Verification items for the finished model (mm, model axes). Face numbers are marked on the shaded views. A direction names the side the tool comes from. Round coordinates to 2 decimals unless told otherwise and drop trailing zeros. Write each loop counter-clockwise with the first axis right and the second up, starting at its lowest first coordinate (ties: lowest second). Pieces come first, ordered by that corner, then holes. Notation, with made-up numbers: M -6,49 L 40,49 A18 cw 40,61 Z; hole C 57.25,71 d7. An arc over 180 degrees is marked long. One line per item, written item: value. Start each with the question number.
Item 1: Gauge pin test, flat ends, axial feed: pin 1 (1.5 mm diameter, centred on y = 6.5, z = 4, fed in from -X); pin 2 (17 mm diameter, centred on x = 0, y = 0, fed in from -Z); pin 3 (4 mm diameter, centred on x = -6, z = 1.5, fed in from +Y). Record the tip position at first contact, or that the pin passes through.
Item 2: Thickness scan on probe 1 along Y at (x, z) = (0, 2.5) (3 decimals); probe 2 along Z at (x, y) = (11, 7.75); probe 3 along Y at (x, z) = (0, -1.85) (3 decimals). Record the ranges inside material, lowest first. Write a range as from..to.
Item 3: Tool access check on the marked faces 1, 2 and 3. Record the directions out of +Z, -Z, +X, -X, +Y, -Y that give a thin tool (end or side, any length) a straight path to the whole face; none if there is none.
Item 4: Section check C-C, the plane z = 2.75. Record the cut outline in (x, y) (3 decimals).
Autodesk Inventor part; units mm, degrees
ref_plane "YZ Plane" through (0, 0, 0) normal (1, 0, 0) x (0, 1, 0)
ref_plane "XZ Plane" through (0, 0, 0) normal (0, 1, 0) x (-1, 0, 0)
ref_plane "XY Plane" through (0, 0, 0) normal (0, 0, 1) x (1, 0, 0)
sketch "Sketch1" plane through (0, 0, 0) normal (0, 0, 1) x (1, 0, 0)
  circle A0 centre (0, 0) radius 9.525
  circle A1 centre (0, 0) radius 12.7
  circle A2 centre (0, 0) radius 14.2875
  dimension "d0" = 19.05
  dimension "d1" = 25.4
  dimension "d2" = 28.575
extrude "Extrusion1" add sketch "Sketch1" along normal blind 4.7625 contours A1
extrude "Extrusion2" add sketch "Sketch1" against normal blind 1.5875 contours A1 | A2
chamfer "Chamfer1" distance 0.254 angle 45 4 edges at (-12.7, 0, 4.7625) (-9.525, 0, 4.7625) (-14.2875, 0, 0) (-14.2875, 0, -1.5875)
sketch "Sketch2" plane through (0, 0, -1.5875) normal (0, 0, -1) x (-1, 0, 0)
  circle A0 centre (0, 0) radius 9.525
  circle A1 centre (0, 0) radius 14.2875
  circle A2 centre (0, 0) radius 10.3188
  dimension "d10" = 20.6375
extrude "Extrusion3" add sketch "Sketch2" along normal blind 0.3969 contours A2
properties part number "Ball Shifting Bushing" material "Brass, Soft Yellow"
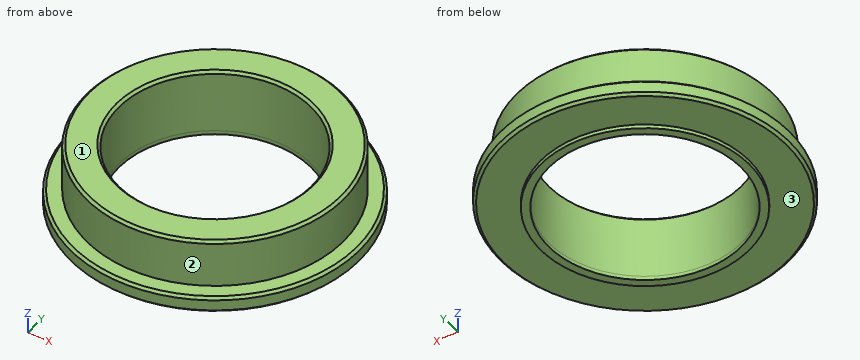
Response values:
1. pin 1: stops at x = -11.32
1. pin 2: passes through
1. pin 3: stops at y = 13.37
2. probe 1: y = -12.7..-9.525, 9.525..12.7
2. probe 2: z = -1.59..0
2. probe 3: y = -10.319..-9.525, 9.525..10.319
3. face 1: +Z, +X, -X, +Y, -Y
3. face 2: +Z
3. face 3: -Z
4. outline: C 0,0 d25.4; hole C 0,0 d19.05
